Verification items for the finished model (mm, model axes). Face numbers are marked on the shaded views. A direction names the side the tool comes from. Give positions to 0.01 mm unless a question says otherwise; leave off trailing zeros. Order: outer loops, then holes, each group sorted by start corner. A loop starts at its lowest first (then second) coordinate and runs counter-clockwise, first axis right, second up. Notation, with made-up numbers: (-34.75, -6) -> (0.25, -6) arc R15 ccw to (0.25, 4) -> close; hole circle Ø9 at (44.25, -16). An arc over 180 degrees is marked (long way). One line per question, with ' | ' between items. Start each with the question number.
Q1. Section check C-C on y = 3.5. Record the cut outline in (x, z), plus the area to 3 significant figures.
Q2. Material ranges on probe 1 along Z at (x, y) = (-1, 7.25); probe 2 along Z at (x, y) = (10.5, 7.75); probe 3 along X at (y, z) = (0.75, 0), recorded low to high. Write a range as [from, to].
Q3. Section check D-D on z = 13.5. Give the number of separate pieces and of enclosed holes in the cut face, plus the area to 3 significant figures.
Q4. Section check A-A on x = -2. Record the cut outline in (y, z).
Q5. Access from +Z, -Z, +X, -X, +Y, -Y to the whole of each face (thin tool, end or side, straight path). Record for the marked faces 1, 2 and 3.
Q6. Mould release check, pull along Z, two halves, no side actions. Record for the marked faces 4, 5 and 6: released by +Z, released by -Z, zero draft, split by the parting line, or undercut.
Q7. Go/stop test with flat-tipped pins: pin 1 (8 mm diameter, centred on x = 6.5, z = -8.5, fed in from -Y); pin 2 (2 mm diameter, centred on x = -4, y = 7, fed in from -Z); pin 3 (1.5 mm diameter, centred on x = -3.5, y = 3, fed in from -Z); pin 4 (5 mm diameter, centred on x = 8, z = 12.5, fed in from +Y). Record where each tip stops, or that it passes through.
Q8. Section check B-B on y = 6. Record the cut outline in (x, z), plus the area to 3 significant figures.
from build123d import *

# Parameters (mm, degrees)
SKETCH_1_R          = 1
EXTRUDE_2_DEPTH     = 9
SKETCH_4_R          = 1
CUT_EXTRUDE_3_DEPTH = 2.5
SKETCH_5_R          = 2.5
CUT_EXTRUDE_4_DEPTH = 5
CUT_EXTRUDE_5_DEPTH = 10


with BuildPart() as part:
    # 草图1 → 凸台-拉伸2 (new body)
    with BuildSketch(Plane(origin=(0, 0, 0), x_dir=(1, 0, 0), z_dir=(0, 1, 0))):
        with BuildLine():
            Line((3.663143512, 20.638777874), (-8.440521732, 12.399902939))
            ThreePointArc((-8.440521732, 12.399902939), (-14.805433948, -2.408137375), (-4.07565223, -14.435686991))
            Line((-4.07565223, -14.435686991), (-3.023376015, -14.692147477))
            Line((-3.023376015, -14.692147477), (11.540736309, -18.241709146))
            ThreePointArc((11.540736309, -18.241709146), (15.964213302, -14.422684135), (12.48297659, -9.728742113))
            Line((12.48297659, -9.728742113), (-3.617537803, -10.389704275))
            ThreePointArc((-3.617537803, -10.389704275), (-10.906788746, -1.440310357), (-6.190548031, 9.094484579))
            Line((-6.190548031, 9.094484579), (5.913117212, 17.333359514))
            Line((5.913117212, 17.333359514), (3.663143512, 20.638777874))
        make_face()
        with Locations(Location((1.196028789, -12.910534794, 0), (0, 0, 270))):
            Circle(SKETCH_1_R, mode=Mode.SUBTRACT)
        with Locations(Location((11.696028789, -13.950268893, 0), (0, 0, 270))):
            Circle(SKETCH_1_R, mode=Mode.SUBTRACT)
    extrude(amount=EXTRUDE_2_DEPTH)

    # 草图4 → 切除-拉伸3 (cut)
    with BuildSketch(Plane(origin=(0, 9, 0), x_dir=(1, 0, 0), z_dir=(0, 1, 0))):
        with BuildLine():
            ThreePointArc((11.696028789, -16.950268893), (14.696028789, -13.950268893), (11.696028789, -10.950268893))
            Line((11.696028789, -10.950268893), (0.791673154, -10.701877185))
            Line((0.791673154, -10.701877185), (0.696028789, -10.69969849))
            ThreePointArc((0.696028789, -10.69969849), (-1.404446611, -12.80017389), (0.696028789, -14.90064929))
            Line((0.696028789, -14.90064929), (11.696028789, -16.950268893))
        make_face()
        with Locations(Location((1.196028789, -12.910534794, 0), (0, 0, 270))):
            Circle(SKETCH_4_R, mode=Mode.SUBTRACT)
        with Locations(Location((11.696028789, -13.950268893, 0), (0, 0, 270))):
            Circle(SKETCH_4_R, mode=Mode.SUBTRACT)
    extrude(amount=-CUT_EXTRUDE_3_DEPTH, mode=Mode.SUBTRACT)

    # 草图5 → 切除-拉伸4 (cut)
    with BuildSketch(Plane(origin=(-8.440521732, 0, -12.399902939), x_dir=(-0.8266601959267582, 0, 0.5627014487899723), z_dir=(-0.5627014487899723, 0, -0.8266601959267582))):
        with Locations((-14.641645144, 4.5)):
            Circle(SKETCH_5_R)
    extrude(amount=-CUT_EXTRUDE_4_DEPTH, mode=Mode.SUBTRACT)

    # 草图6 → 切除-拉伸5 (cut)
    with BuildSketch(Plane(origin=(-3.549514122, 0, 14.563917234), x_dir=(0.9715611869561729, 0, 0.23678863993087312), z_dir=(-0.23678863993087312, 0, 0.9715611869561729))):
        with BuildLine():
            Line((-0.541538829, 4.5), (18.960921895, 4.5))
            Line((18.960921895, 4.5), (18.960921895, 0))
            Line((18.960921895, 0), (-0.541538829, 0))
            Line((-0.541538829, 0), (-5.041538829, 0))
            ThreePointArc((-5.041538829, 0), (-1.859558314, 1.318019485), (-0.541538829, 4.5))
        make_face()
    extrude(amount=-CUT_EXTRUDE_5_DEPTH, mode=Mode.SUBTRACT)


solid = part.part
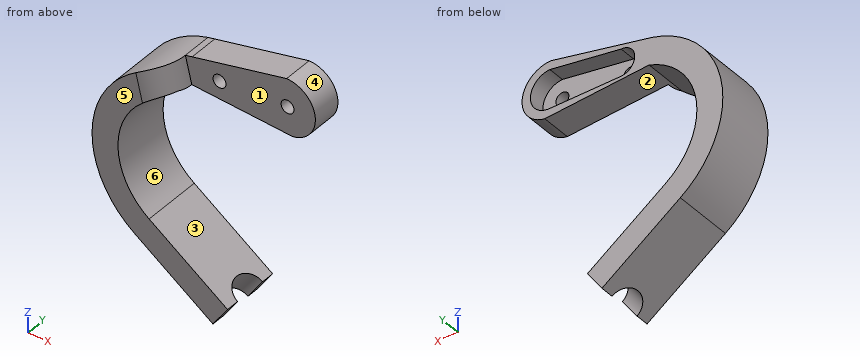
Filled in:
1) outline: (-8.44, -12.4) -> (1.77, -19.35) -> (4.02, -16.04) -> (-6.19, -9.09) arc R11 cw to (-3.62, 10.39) -> (-3.2, 10.37) -> (-4.18, 14.4) arc R15 ccw to start | area: 167 mm²
2) probe 1: [-17.46, -12.63], [10.28, 11.56], [14.04, 15.19] | probe 2: [9.81, 10.92], [16.73, 17.99] | probe 3: [-15, -11]
3) separate pieces: 3 | enclosed holes: 0 | area: 62.5 mm²
4) outline: (0, -16.78) -> (9, -16.78) -> (9, -11.95) -> (0, -11.95) -> close; (4.5, 10.32) -> (9, 10.32) -> (9, 14.94) -> (4.5, 14.94) -> close
5) face 1: +Z, +X, -Y | face 2: +Y, -Y | face 3: +X, +Y, -Y
6) face 4: split by the parting line | face 5: zero draft | face 6: undercut
7) pin 1: through | pin 2: z = -16.1 | pin 3: z = -16.27 | pin 4: y = 9
8) outline: (-8.44, -12.4) -> (2.01, -19.51) -> (4.26, -16.21) -> (-6.19, -9.09) arc R11 cw to (-3.62, 10.39) -> (12.48, 9.73) arc R4.29 ccw to (11.54, 18.24) -> (-4.08, 14.44) arc R15 ccw to start; hole circle Ø2 at (1.2, 12.91); hole circle Ø2 at (11.7, 13.95) | area: 288 mm²
